Here's how the part is built. I have some questions about the finished solid (model axes, mm). Face numbers are marked on the shaded views. A direction names the side the tool comes from. Coordinates: 2 decimals unless noted, no trailing zeros. Loops run counter-clockwise (first coordinate to the right, second up) from the corner with the lowest first, then second, coordinate; pieces in that order, holes last. Notation, with made-up numbers: M 73.5,21.5 L 83.5,21.5 A31 cw 83.5,59.5 Z; hole C 22,77.5 d11. An arc over 180 degrees is marked long. Use CSV: the item, a comma, the result in double quotes. Start each with the question number.
Q1. If we mould it in two halves opening along Y, with no side actions, what happens to the marked faces 1, 2, 3 and 4? For each: +Y half, -Y half, draft (parallel to the pull), parting line (faces both ways), or undercut.
Q2. If we section it at A-A (x = -22): Please give me the cut outline in (y, z), and give its area (3 significant figures).
Q3. For pin 1 Ø9.5 at (y, z) = (5.5, 11.5) entering from -X; pin 2 Ø0.9 at (x, z) = (-28.5, 23.5) entering from -Y; pin 3 Ø1 at (x, z) = (-21, 8.5) entering from +Y; pin 4 Ø10 at (x, z) = (74.5, 22) entering from +Y, each with a flat end and sliding along its axis, tell me the tip position at first contact or that it passes through.
Q4. Please list where these lines run through material, in increasing order: probe 1 along Y at (x, z) = (-22, 3.25); probe 2 along Y at (x, z) = (-30, 1.5); probe 3 along X at (y, z) = (15.5, 5.25). Write a range as [from, to].
Q5. If we section it at D-D (x = 8): Please give me the cut outline in (y, z).
Q6. Which directions (+Z, -Z, +X, -X, +Y, -Y) give clear straight access to the entire face, cutting with the end or side of a thin tool? Please do the marked faces 5, 6 and 7.
Q7. If we section it at C-C (y = -12): State how many separate pieces and enclosed holes the cut face has, and give its area (3 significant figures).
Q8. If we section it at B-B (y = 17.5): Please give me the cut outline in (x, z).
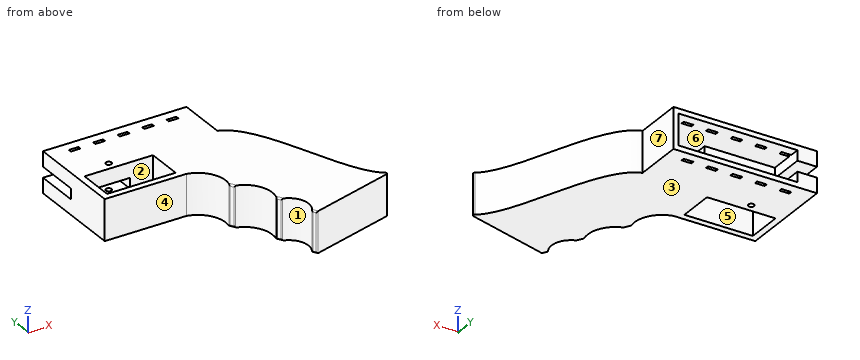
from build123d import *

# Parameters (mm, degrees)
F0_W     = 42
F0_H     = 22
F0_W_2   = 6
F0_H_2   = 2
F1_DEPTH = 25
F2_W     = 30
F2_H     = 19
F2_W_2   = 20
F2_H_2   = 6.5
F2_W_3   = 12
F3_DEPTH = 22
F4_DEPTH = 55
F5_DEPTH = 34
F6_DEPTH = 27
F7_R     = 1
F8_R     = 1.75
F9_DEPTH = 25.0010001


with BuildPart() as f1:
    # F0 (on Top) → F1 (new body)
    with BuildSketch(Plane.XY):
        Polygon((44, 30), (-44, 30), (-44, -30), (6, -30), (44, -30), (44, 0), align=None)
        with Locations((-19, -15)):
            Rectangle(F0_W, F0_H, mode=Mode.SUBTRACT)
        with Locations((-29, 23)):
            Rectangle(F0_W_2, F0_H_2, mode=Mode.SUBTRACT)
        with Locations((-14, 23)):
            Rectangle(F0_W_2, F0_H_2, mode=Mode.SUBTRACT)
        with Locations((1, 23)):
            Rectangle(F0_W_2, F0_H_2, mode=Mode.SUBTRACT)
        with Locations((16, 23)):
            Rectangle(F0_W_2, F0_H_2, mode=Mode.SUBTRACT)
        with Locations((31, 23)):
            Rectangle(F0_W_2, F0_H_2, mode=Mode.SUBTRACT)
        with BuildLine():
            add(Edge.make_bspline(
                [(44, 0), (67.8392201662, -7.6675033197), (76.1326849461, -76.210565865), (96, -85)],
                knots=[0, 0, 0, 0, 99.6443676281, 99.6443676281, 99.6443676281, 99.6443676281], degree=3))
            Line((44, 0), (44, -30))
            Line((44, -30), (6, -30))
            ThreePointArc((6, -30), (17.1808031069, -37.8263151446), (19.0039282867, -51.3517645433))
            Line((19.0039282867, -51.3517645433), (20.5282030185, -53.9356737024))
            ThreePointArc((20.5282030185, -53.9356737024), (31.2549165387, -62.3736345883), (32.3205438236, -75.9797363573))
            Line((32.3205438236, -75.9797363573), (33.8448185554, -78.5636455164))
            ThreePointArc((33.8448185554, -78.5636455164), (42.2422484339, -86.1981187462), (40.5220414274, -97.416090841))
            Line((40.5220414274, -97.416090841), (42.0463161591, -100))
            Line((42.0463161591, -100), (96, -85))
        make_face()
    extrude(amount=F1_DEPTH)

    # F2 (on face) → F3 (cut)
    with BuildSketch(Plane(origin=(0, 30, 0), x_dir=(-1, 0, 0), z_dir=(0, 1, 0))):
        Polygon((32, 22), (-11, 22), (-11, 3), (32, 3), (32, 9.25), (12, 9.25), (12, 15.75), (32, 15.75), align=None)
        with Locations((-26, 12.5)):
            Rectangle(F2_W, F2_H)
        with Locations((22, 12.5)):
            Rectangle(F2_W_2, F2_H_2)
        with Locations((38, 12.5)):
            Rectangle(F2_W_3, F2_H_2)
    extrude(amount=-F3_DEPTH, mode=Mode.SUBTRACT)

    # F2 (on face) → F4 (cut)
    with BuildSketch(Plane(origin=(0, 30, 0), x_dir=(-1, 0, 0), z_dir=(0, 1, 0))):
        with Locations((-26, 12.5)):
            Rectangle(F2_W, F2_H)
    extrude(amount=-F4_DEPTH, mode=Mode.SUBTRACT)

    # F2 (on face) → F5 (cut, through all)
    with BuildSketch(Plane(origin=(0, 30, 0), x_dir=(-1, 0, 0), z_dir=(0, 1, 0))):
        with Locations((22, 12.5)):
            Rectangle(F2_W_2, F2_H_2)
    extrude(amount=-F5_DEPTH, mode=Mode.SUBTRACT)

    # F2 (on face) → F6 (cut)
    with BuildSketch(Plane(origin=(0, 30, 0), x_dir=(-1, 0, 0), z_dir=(0, 1, 0))):
        with Locations((38, 12.5)):
            Rectangle(F2_W_3, F2_H_2)
    extrude(amount=-F6_DEPTH, mode=Mode.SUBTRACT)

    # F7
    f7_edges = [f1.edges().sort_by_distance(p)[0] for p in [
        (20.528203, -53.935674, 12.5),
        (19.003928, -51.351765, 12.5),
        (19.766066, -52.643719, 0),
        (19.766066, -52.643719, 25),
        (33.844819, -78.563646, 12.5),
        (32.320544, -75.979736, 12.5),
        (33.082681, -77.271691, 0),
        (33.082681, -77.271691, 25),
        (42.046316, -100, 12.5),
        (40.522041, -97.416091, 12.5),
        (41.284179, -98.708045, 0),
        (41.284179, -98.708045, 25),
        (96, -85, 12.5),
    ]]
    fillet(f7_edges, radius=F7_R)

    # F8 (on face) → F9 (cut, through all)
    with BuildSketch(Plane.XY.offset(25)):
        with Locations((-22, 1)):
            Circle(F8_R)
    extrude(amount=-F9_DEPTH, mode=Mode.SUBTRACT)


solid = f1.part
Results below:
1,face 1,"undercut"
1,face 2,"undercut"
1,face 3,"draft"
1,face 4,"-Y half"
2,outline,"M -30,0 L -26,0 L -26,25 L -30,25 Z; M -4,0 L -0.75,0 L -0.75,9.25 L -4,9.25 Z; M -4,15.75 L -0.75,15.75 L -0.75,25 L -4,25 Z; M 2.75,0 L 30,0 L 30,3 L 8,3 L 8,9.25 L 2.75,9.25 Z; M 2.75,15.75 L 8,15.75 L 8,22 L 30,22 L 30,25 L 2.75,25 Z"
2,area,"389 mm^2"
3,pin 1,"x = -44"
3,pin 2,"y = -30"
3,pin 3,"y = 8"
3,pin 4,"y = -37.06"
4,probe 1,"[-30, -26], [-4, -0.75], [2.75, 8]"
4,probe 2,"[-30, -26], [-4, 22], [24, 30]"
4,probe 3,"[-44, -32], [41, 44]"
5,outline,"M -30.53,0 L 30,0 L 30,3 L 8,3 L 8,22 L 30,22 L 30,25 L -30.53,25 Z"
6,face 5,"+Z, -Z"
6,face 6,"+Y"
6,face 7,"+Z, -Z, +X, +Y"
7,separate pieces,"2"
7,enclosed holes,"1"
7,area,"914 mm^2"
8,outline,"M -44,0 L 44,0 L 44,25 L -44,25 L -44,15.75 L -32,15.75 L -32,22 L 41,22 L 41,3 L -32,3 L -32,9.25 L -44,9.25 Z"
